```python
from build123d import *

# Parameters (mm, degrees)
F0_W      = 31.75
F0_H      = 101.6
F1_DEPTH  = 1.524
F2_W      = 31.75
F2_H      = 4.1754661679
F3_DEPTH  = 0.508
F5_W      = 31.75
F5_H      = 51.593744238
F6_DEPTH  = 1.27
F8_DEPTH  = 1.27
F10_DEPTH = 0.254
F12_DEPTH = 0.254


with BuildPart() as f1:
    # F0 (on Front) → F1 (new body)
    with BuildSketch(Plane.XZ):
        with Locations((-13.0295728195, 11.8000358343)):
            Rectangle(F0_W, F0_H)
    extrude(amount=F1_DEPTH)

    # F2 (on face) → F3 (join)
    with BuildSketch(Plane.XZ.offset(1.524)):
        with Locations((-13.0295728195, 60.5123027503)):
            Rectangle(F2_W, F2_H)
    extrude(amount=F3_DEPTH)

    # F5 (on offset) → F6 (join)
    with BuildSketch(Plane.XZ.offset(2.032)):
        with Locations((-12.9512589192, 36.5513293073)):
            Rectangle(F5_W, F5_H)
    extrude(amount=F6_DEPTH)

    # F7 (on face) → F8 (cut)
    with BuildSketch(Plane.XZ.offset(3.302)):
        Polygon((-13.2123797666, 54.7112040222), (-22.1023797666, 54.7112040222), (-22.1023797666, 16.5791511536), (-4.3223797666, 16.5791511536), (-4.3223797666, 25.4691511536), (-13.2123797666, 25.4691511536), align=None)
    extrude(amount=-F8_DEPTH, mode=Mode.SUBTRACT)

    # F9 (on face) → F10 (cut)
    with BuildSketch(Plane(origin=(0, 0, 0), x_dir=(-1, 0, 0), z_dir=(0, 1, 0))):
        with BuildLine():
            Line((4.9357393071, 26.6371323704), (17.3911272623, 40.1263655171))
            ThreePointArc((17.3911272623, 40.1263655171), (6.031549564, 38.1203135447), (4.9357393071, 26.6371323704))
        make_face()
        with BuildLine():
            ThreePointArc((8.9218471858, 23.0649033911), (18.1089201368, 23.6009763334), (22.5545728195, 31.6586345434))
            ThreePointArc((22.5545728195, 31.6586345434), (22.1499463329, 34.405343843), (20.9704443205, 36.9186901328))
            Line((20.9704443205, 36.9186901328), (8.9218471858, 23.0649033911))
        make_face()
    extrude(amount=-F10_DEPTH, mode=Mode.SUBTRACT)

    # F11 (on face) → F12 (cut)
    with BuildSketch(Plane(origin=(0, 0, 0), x_dir=(-1, 0, 0), z_dir=(0, 1, 0))):
        with BuildLine():
            Line((14.8511272623, 46.0878358148), (11.4618471858, 46.0878358148))
            Line((11.4618471858, 46.0878358148), (11.4618471858, 41.0537322724))
            ThreePointArc((11.4618471858, 41.0537322724), (13.1585452479, 41.1827613335), (14.8511272623, 41.0078358148))
            Line((14.8511272623, 41.0078358148), (14.8511272623, 46.0878358148))
        make_face()
        Polygon((14.8511272623, 37.3755357304), (11.4618471858, 33.7049323485), (11.4618471858, 25.9854606917), (14.8511272623, 29.8825420583), align=None)
        with BuildLine():
            ThreePointArc((14.8511272623, 41.0078358148), (13.1585452479, 41.1827613335), (11.4618471858, 41.0537322724))
            Line((11.4618471858, 41.0537322724), (11.4618471858, 33.7049323485))
            Line((11.4618471858, 33.7049323485), (14.8511272623, 37.3755357304))
            Line((14.8511272623, 37.3755357304), (14.8511272623, 41.0078358148))
        make_face()
        with BuildLine():
            Line((14.8511272623, 29.8825420583), (11.4618471858, 25.9854606917))
            Line((11.4618471858, 25.9854606917), (11.4618471858, 22.2635368144))
            ThreePointArc((11.4618471858, 22.2635368144), (13.1585452479, 22.1345077534), (14.8511272623, 22.3094332721))
            Line((14.8511272623, 22.3094332721), (14.8511272623, 29.8825420583))
        make_face()
        with BuildLine():
            ThreePointArc((14.8511272623, 22.3094332721), (13.1585452479, 22.1345077534), (11.4618471858, 22.2635368144))
            Line((11.4618471858, 22.2635368144), (11.4618471858, 17.1835368144))
            Line((11.4618471858, 17.1835368144), (14.8511272623, 17.1835368144))
            Line((14.8511272623, 17.1835368144), (14.8511272623, 22.3094332721))
        make_face()
    extrude(amount=-F12_DEPTH, mode=Mode.SUBTRACT)


solid = f1.part
```
Input: part model. Units: mm. Frame: model coordinates. A direction names the side the tool comes from. Give positions to 0.01 mm unless a question says otherwise; leave off trailing zeros. Order: outer loops, then holes, each group sorted by start corner. A loop starts at its lowest first (then second) coordinate and runs counter-clockwise, first axis right, second up.
1. Mould query, pull axis Y, two halves, no side actions, for faces 1 (the flat face through (-13, -1.524, 10)), 2 (the flat face through (-13, 0, 13)), 3 (the flat face through (-28.905, -1, 11)), 4 (the flat face through (-13, -3.302, 37)). Classes: released by +Y, released by -Y, zero draft, split by the parting line, or undercut.
Derived:
face 1: undercut
face 2: released by +Y
face 3: zero draft
face 4: released by -Y
2. Reachability of faces 5 (the flat face through (2.845, -1, 11)), 6 (the flat face through (-13, -1, 62.6)) from +Z, -Z, +X, -X, +Y, -Y: full face, straight path, thin tool, end or side. Return the list, or none.
Derived:
face 5: +Z, -Z, +X, +Y
face 6: +Z, +X, -X, +Y, -Y
3. Material intervals for L1, parallel to Z at x = -7.5, y = -2.85; L2, parallel to Y at x = 2, z = 54; L3, parallel to X at y = -2.15, z = 32.5, sorted ascending.
Derived:
L1: z = 10.75 to 16.58, 25.47 to 62.35
L2: y = -3.3 to -2.03, -1.52 to 0
L3: x = -28.83 to -22.1, -13.21 to 2.92
4. Section D-D on z = -2.5. Return the cut outline in (x, y), and give its area (3 significant figures).
Derived:
outline: (-28.9, -1.52) - (2.85, -1.52) - (2.85, 0) - (-28.9, 0) - close
area: 48.4 mm2
5. Section B-B on x = -8. Return the cut outline in (y, z), and give its area (3 significant figures).
Derived:
outline: (-3.3, 10.75) - (-2.03, 10.75) - (-2.03, 16.58) - (-3.3, 16.58) - close; (-3.3, 25.47) - (-2.03, 25.47) - (-2.03, 58.42) - (-1.52, 58.42) - (-1.52, -39) - (0, -39) - (0, 29.96) - (-0.25, 29.96) - (-0.25, 39.75) - (0, 39.75) - (0, 62.6) - (-2.03, 62.6) - (-2.03, 62.35) - (-3.3, 62.35) - close
area: 209 mm2
6. Pin query (flat end, axial travel): pin 1 (0.6 mm diameter, centred on y = -2.5, z = 23, fed in from -X); pin 2 (0.6 mm diameter, centred on y = -0.5, z = -1, fed in from +X). Return the tip coordinate at first contact, or that it passes through.
Derived:
pin 1: stops at x = -28.83
pin 2: stops at x = 2.85
7. Section C-C on x = -2. Return the cut outline in (y, z).
Derived:
outline: (-3.3, 10.75) - (-2.03, 10.75) - (-2.03, 58.42) - (-1.52, 58.42) - (-1.52, -39) - (0, -39) - (0, 62.6) - (-2.03, 62.6) - (-2.03, 62.35) - (-3.3, 62.35) - close
8. Section A-A on y = -2.55. Return the cut outline in (x, z).
Derived:
outline: (-28.83, 10.75) - (2.92, 10.75) - (2.92, 62.35) - (-28.83, 62.35) - close; hole (-22.1, 16.58) - (-4.32, 16.58) - (-4.32, 25.47) - (-13.21, 25.47) - (-13.21, 54.71) - (-22.1, 54.71) - close
